Answer from the drawing. Dimensions are ordinates in mm from the lowest x, y and z of the part. Give positions to 0.01 mm unless a question says otherwise; leave off trailing zeros. Loops run counter-clockwise (first coordinate to the right, second up) from the corner with the lowest first, then second, coordinate; pieces in that order, holes last. Notation, with made-up numbers: (-26, 18.5) -> (5, 18.5) arc R13 ccw to (5, 35.5) -> close; hole circle Ø11 at (34.5, 9). An arc over 180 degrees is marked (long way). Answer as CSV lines item,"result". Start each with the question number.
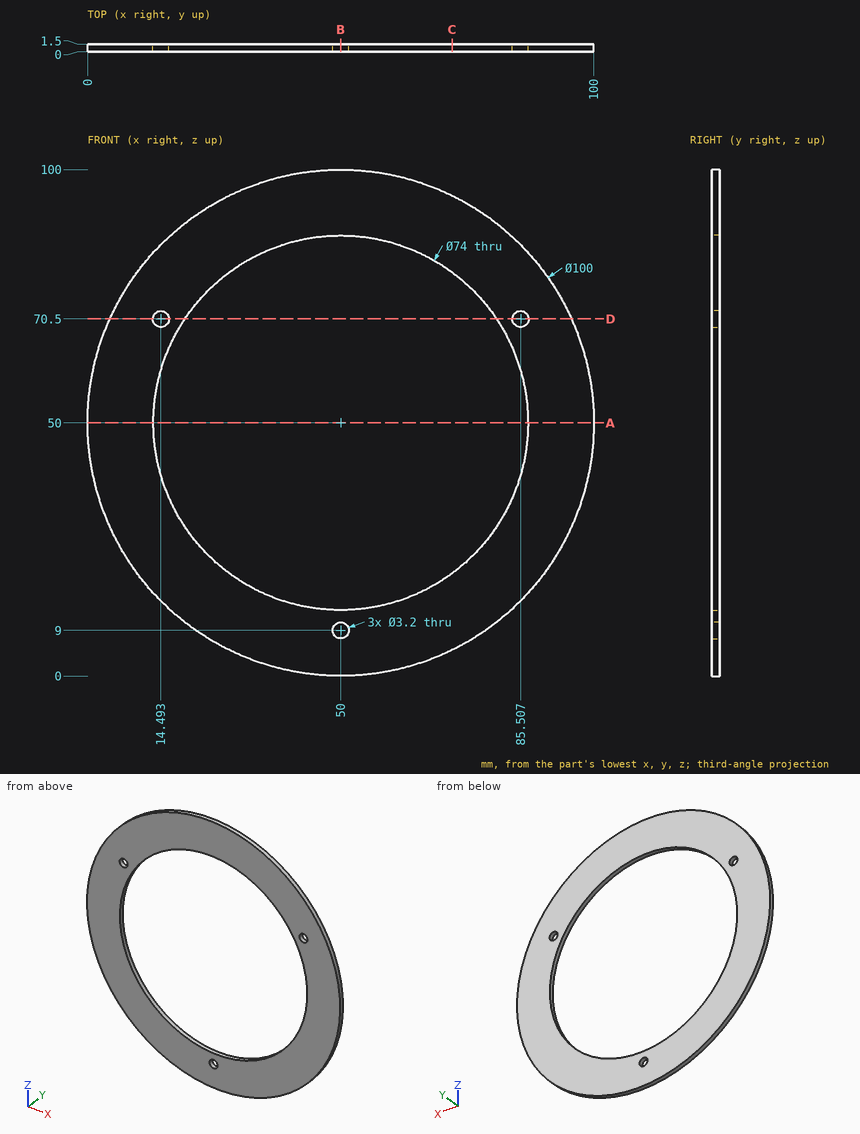
(1) Find section C-C on x = 72. Write down the section's boundary in (y, z).
(2) Find the intervals of material crossed by line 1 along X through (y, z) = (1, 70.5); line 2 along Z through (x, y) = (49.5, 0.95); line 3 along X through (y, z) = (1.4, 25), in increasing order. Write a range as from..to.
(3) Find section A-A on z = 50. Write down the section's boundary in (x, y), then the cut area to 3 significant figures.
(4) Find section B-B on x = 50. Write down the section's boundary in (y, z), then the cut area to 3 significant figures.
(5) Find section D-D on z = 70.5. Write down the section's boundary in (x, y), then the cut area to 3 significant figures.
(6) This flat-tipped pin is pushed along its axis until it touches: P1, Ø3, axis at x = 85.51, z = 70.5, coming from the +Y side (1 decimal). Where does it stop, or does it pass through?
Answer block:
1,outline,"(0, 5.1) -> (1.5, 5.1) -> (1.5, 20.25) -> (0, 20.25) -> close; (0, 79.75) -> (1.5, 79.75) -> (1.5, 94.9) -> (0, 94.9) -> close"
2,line 1,"x = 4.4..12.89, 16.09..19.2, 80.8..83.91, 87.11..95.6"
2,line 2,"z = 0..7.48, 10.52..13, 87..100"
2,line 3,"x = 6.7..22.72, 77.28..93.3"
3,outline,"(0, 0) -> (13, 0) -> (13, 1.5) -> (0, 1.5) -> close; (87, 0) -> (100, 0) -> (100, 1.5) -> (87, 1.5) -> close"
3,area,"39.0 mm2"
4,outline,"(0, 0) -> (1.5, 0) -> (1.5, 7.4) -> (0, 7.4) -> close; (0, 10.6) -> (1.5, 10.6) -> (1.5, 13) -> (0, 13) -> close; (0, 87) -> (1.5, 87) -> (1.5, 100) -> (0, 100) -> close"
4,area,"34.2 mm2"
5,outline,"(4.4, 0) -> (12.89, 0) -> (12.89, 1.5) -> (4.4, 1.5) -> close; (16.09, 0) -> (19.2, 0) -> (19.2, 1.5) -> (16.09, 1.5) -> close; (80.8, 0) -> (83.91, 0) -> (83.91, 1.5) -> (80.8, 1.5) -> close; (87.11, 0) -> (95.6, 0) -> (95.6, 1.5) -> (87.11, 1.5) -> close"
5,area,"34.8 mm2"
6,P1,"passes through"
